Model file for the job. Use its own axes, mm. Face numbers are marked on the shaded views. Round coordinates to 2 decimals unless told otherwise and drop trailing zeros. Order: outer loops, then holes, each group sorted by start corner. A loop starts at its lowest first (then second) coordinate and runs counter-clockwise, first axis right, second up. Notation, with made-up numbers: M -12,31.25 L 2,31.25 A20 ccw 2,48.25 Z; hole C 87,26.25 d2. An arc over 180 degrees is marked long. Return JSON: item names as keys, results as strings. Group by question number.
Item 1: Slice it at C-C on z = 15. Write the cut outline in (x, y) (3 decimals).
Item 2: Pin check, flat tips, straight feed: pin 1 Ø9.5 at (x, z) = (13.5, 0) entering from -Y; pin 2 Ø0.8 at (x, y) = (10.5, -4) entering from +Z; pin 3 Ø1.6 at (x, y) = (-10, -2) entering from -Z. Stop position of each tip, or through.
Item 3: Slice it at A-A on y = -4.5. Write the cut outline in (x, z).
Item 4: Probe line 1 along Z through (x, y) = (-8, -0.25); line 2 along Z through (x, y) = (-11, 0.75); line 3 along X through (y, z) = (-2, -14.5). List the from-to ranges inside material, lowest first.
Item 5: Slice it at B-B on y = -0.75. Give the number of separate pieces and of enclosed holes in the cut face, then the cut area to 3 significant figures.
Item 6: Pull direction X, two halves, no side cores. Call the marked faces 1 and 2: pulls with the +X half, pulls with the -X half, needs draft (parallel to the pull), parting line crosses it, or undercut.
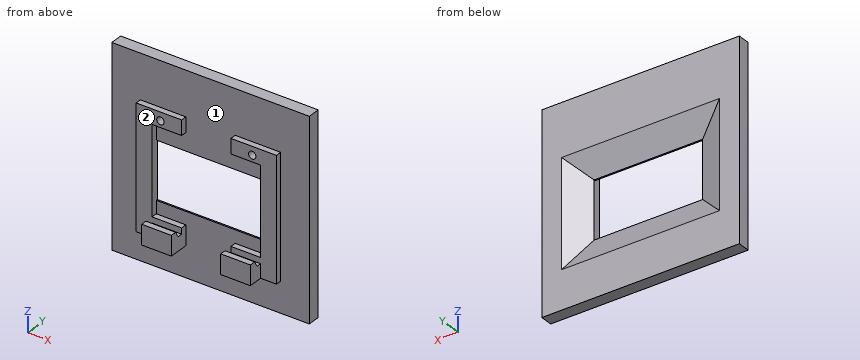
Autodesk Inventor part; units mm, degrees
ref_plane "YZ Plane" through (0, 0, 0) normal (1, 0, 0) x (0, 1, 0)
ref_plane "XZ Plane" through (0, 0, 0) normal (0, 1, 0) x (-1, 0, 0)
ref_plane "XY Plane" through (0, 0, 0) normal (0, 0, 1) x (1, 0, 0)
sketch "Sketch1" plane through (0, 0, 0) normal (0, 1, 0) x (-1, 0, 0)
  line L0 (-25.4, 25.4) -> (25.4, 25.4)
  line L1 (25.4, 25.4) -> (25.4, -25.4)
  line L2 (25.4, -25.4) -> (-25.4, -25.4)
  line L3 (-25.4, -25.4) -> (-25.4, 25.4)
  line L4 (-25.4, 25.4) -> (25.4, -25.4) construction
  line L5 (25.4, 25.4) -> (-25.4, -25.4) construction
  point P0 (0, 0)
  dimension "d0" = 50.8
  dimension "d1" = 50.8
extrude "Extrusion1" add sketch "Sketch1" along normal blind 3.175
sketch "Sketch2" plane through (0, 0, 0) normal (0, -1, 0) x (1, 0, 0)
  line L0 (-11.811, 11.811) -> (11.811, 11.811) construction
  line L1 (11.811, 11.811) -> (11.811, -11.811) construction
  line L2 (11.811, -11.811) -> (-11.811, -11.811) construction
  line L3 (-11.811, -11.811) -> (-11.811, 11.811) construction
  circle A0 centre (-11.811, 11.811) radius 0.9525
  line L4 (13.97, 13.97) -> (-13.97, 13.97) construction
  line L5 (-13.97, 13.97) -> (-13.97, -13.97) construction
  line L6 (-13.97, -13.97) -> (13.97, -13.97) construction
  line L7 (13.97, -13.97) -> (13.97, 13.97) construction
  line L8 (13.97, 13.97) -> (6.35, 13.97)
  line L9 (6.35, 13.97) -> (6.35, 10.16)
  line L10 (6.35, 10.16) -> (13.97, 10.16)
  line L11 (13.97, 10.16) -> (13.97, 13.97)
  line L12 (-13.97, 13.97) -> (-6.35, 13.97)
  line L13 (-6.35, 13.97) -> (-6.35, 10.16)
  line L14 (-6.35, 10.16) -> (-13.97, 10.16)
  line L15 (-13.97, 10.16) -> (-13.97, 13.97)
  circle A1 centre (11.811, 11.811) radius 0.9525
  line L16 (13.97, 13.97) -> (18.034, 13.97)
  line L17 (18.034, 13.97) -> (18.034, -17.526)
  line L18 (18.034, -17.526) -> (13.97, -17.526)
  line L19 (13.97, -17.526) -> (13.97, 13.97)
  line L20 (-13.97, 13.97) -> (-18.034, 13.97)
  line L21 (-18.034, 13.97) -> (-18.034, -17.526)
  line L22 (-18.034, -17.526) -> (-13.97, -17.526)
  line L23 (-13.97, -17.526) -> (-13.97, 13.97)
  point P0 (0, 0)
  point P1 (11.811, 0)
  point P2 (0, 11.811)
  point P3 (0, -13.97)
  point P4 (-13.97, 0)
  point P5 (-13.97, 10.16)
  point P6 (13.97, 10.16)
  dimension "d4" = 23.622
  dimension "d5" = 23.622
  dimension "d27" = 27.94
  dimension "d28" = 27.94
  dimension "d29" = 7.62
  dimension "d30" = 3.81
  dimension "d31" = 1.905
  dimension "d32" = 4.064
  dimension "d33" = 4.064
  dimension "d46" = 31.496
extrude "Extrusion2" add sketch "Sketch2" along normal blind 1.524
sketch "Sketch3" plane through (0, 0, 0) normal (0, -1, 0) x (1, 0, 0)
  line L0 (13.97, 13.97) -> (-13.97, 13.97) construction
  line L1 (-13.97, 13.97) -> (-13.97, -13.97) construction
  line L2 (-13.97, -13.97) -> (13.97, -13.97) construction
  line L3 (13.97, -13.97) -> (13.97, 13.97) construction
  line L4 (13.97, 13.97) -> (-13.97, -13.97) construction
  line L5 (-13.97, 13.97) -> (13.97, -13.97) construction
  line L6 (13.97, 5.588) -> (-13.97, 5.588)
  line L7 (-13.97, 5.588) -> (-13.97, -9.144)
  line L8 (-13.97, -9.144) -> (13.97, -9.144)
  line L9 (13.97, -9.144) -> (13.97, 5.588)
  point P0 (0, 0)
  dimension "d18" = 27.94
  dimension "d19" = 27.94
  dimension "d20" = 4.826
  dimension "d21" = 14.732
sketch "Sketch4" plane through (0, 3.175, 0) normal (0, 1, 0) x (1, 0, 0)
  line L0 (-13.97, 9.144) -> (13.97, 9.144)
  line L1 (13.97, -5.588) -> (-13.97, -5.588)
  line L2 (-13.97, -5.588) -> (-13.97, 9.144)
  line L3 (13.97, 9.144) -> (13.97, -5.588)
  line L4 (-20.32, -11.938) -> (20.32, -11.938)
  line L5 (20.32, -11.938) -> (20.32, 15.494)
  line L6 (20.32, 15.494) -> (-20.32, 15.494)
  line L7 (-20.32, 15.494) -> (-20.32, -11.938)
  point P0 (0, 0)
  dimension "d22" = 6.35
sketch "Sketch5" plane through (0, 0, 0) normal (1, 0, 0) x (0, 1, 0)
  line L0 (0, 25.4) -> (0, -25.4)
  line L1 (0, -12.446) -> (-1.524, -12.446)
  line L2 (-1.524, 10.16) -> (-1.524, -17.526)
  line L3 (-1.524, -12.446) -> (-1.524, -13.97)
  line L4 (-1.524, -13.97) -> (-2.794, -13.97)
  line L5 (-2.794, -13.97) -> (-3.6739, -12.446)
  line L6 (-3.6739, -12.446) -> (-5.1979, -12.446)
  line L7 (-5.1979, -12.446) -> (-5.1979, -17.526)
  line L8 (-5.1979, -17.526) -> (0, -17.526)
  line L9 (0, -17.526) -> (0, -12.446)
  line L10 (3.175, -16.002) -> (3.175, 11.43)
  line L11 (0, 13.97) -> (-1.524, 13.97)
  point P0 (0, 0)
  point P1 (0, -17.526)
  dimension "d34" = 1.524
  dimension "d35" = 1.524
  dimension "d36" = 1.27
  dimension "d37" = 120
  dimension "d38" = 1.524
  dimension "d39" = 5.08
  dimension "d40" = 27.94
extrude "Extrusion3" add sketch "Sketch5" along normal mid plane 27.94
sketch "Sketch6" plane through (0, 0, 0) normal (0, -1, 0) x (1, 0, 0)
  line L0 (-13.97, -17.526) -> (13.97, -17.526)
  line L1 (13.97, -12.446) -> (13.97, -17.526)
  line L2 (-13.97, -12.446) -> (13.97, -12.446)
  line L3 (-13.97, -17.526) -> (-13.97, -12.446)
  line L4 (-6.35, -12.446) -> (6.35, -12.446)
  line L5 (6.35, -12.446) -> (6.35, -17.526)
  line L6 (6.35, -17.526) -> (-6.35, -17.526)
  line L7 (-6.35, -17.526) -> (-6.35, -12.446)
  point P0 (0, 0)
  point P1 (0, -12.446)
  point P2 (0, -12.446)
  dimension "d43" = 12.7
extrude "Extrusion4" cut sketch "Sketch6" along normal up to surface (5.1979 mm away) contours L7 L2 L5 L0
sketch "Sketch7" plane through (0, 0, 0) normal (0, -1, 0) x (1, 0, 0)
  circle A0 centre (11.811, 11.811) radius 0.9525
  circle A1 centre (-11.811, 11.811) radius 0.9525
  point P0 (0, 0)
extrude "Extrusion5" cut sketch "Sketch7" against normal blind 2.54
extrude "Extrusion7" cut sketch "Sketch3" against normal blind 0.381
loft "Loft2" cut profiles "Sketch4" section 1 edges at (-13.97, 0.381, -1.778) (0, 0.381, -9.144) (13.97, 0.381, -1.778) (0, 0.381, 5.588) contours L0 L3 L1 L2 | L7 L6 L5 L4
properties part number "DisplayInsert"
Output values:
{
 "1": {"outline": "M -25.4,0 L 25.4,0 L 25.4,3.175 L -25.4,3.175 Z"},
 "2": {"pin 1": "y = -1.52", "pin 2": "z = -12.45", "pin 3": "z = -17.53"},
 "3": {"outline": "M -13.97,-17.53 L -6.35,-17.53 L -6.35,-12.45 L -13.97,-12.45 Z; M 6.35,-17.53 L 13.97,-17.53 L 13.97,-12.45 L 6.35,-12.45 Z"},
 "4": {"line 1": "-17.53 to -12.45, 10.16 to 13.97", "line 2": "-25.4 to -9.98, 6.43 to 11.31, 12.31 to 25.4", "line 3": "-13.97 to -6.35, 6.35 to 13.97"},
 "5": {"separate pieces": "2", "enclosed holes": "2", "area": "386 mm²"},
 "6": {"face 1": "undercut", "face 2": "needs draft"}
}
